Input: part model. Units: mm. Frame: model coordinates. A direction names the side the tool comes from. Coordinates: 2 decimals unless noted, no trailing zeros. Order: outer loops, then holes, each group sorted by start corner. A loop starts at its lowest first (then second) coordinate and runs counter-clockwise, first axis right, second up. Notation, with made-up numbers: (26, 17.5) - (50, 17.5) arc R23 ccw to (50, 49.5) - close; hole circle Ø9 at (58, 78.5). An arc over 180 degrees is marked (long way). Answer as CSV lines item,"result". Start each with the question number.
Item 1: Section B-B (y = -34.8). Output: boundary loops of the cut face in (x, z), and give its area (3 significant figures).
Item 2: Section A-A (z = -27.5). Output: boundary loops of the cut face in (x, y), and give its area (3 significant figures).
Item 3: Access query for faces 5 (the cylindrical face through (-27.903, 27.841, -38.594)), 6 (the cylindrical face through (-27.841, -27.903, -38.594)), 7 (the flat face through (37, 26.7, -39)), 8 (the flat face through (37, -26.7, -39)). Directions: +Z, -Z, +X, -X, +Y, -Y. A direction counts if a zero-diameter tool reaches every point of the face in a straight line with its end or side. Return the directions, or none.
Item 4: Section D-D (y = 0). Output: boundary loops of the cut face in (x, z).
Item 5: Draft query along Y for faces 1 (the cylindrical face through (-41.697, 41.759, -4.93)), 2 (the cylindrical face through (-38.022, -34.377, -5.07)), 3 (the cylindrical face through (6.466, 2.681, 16.587)), 4 (the flat face through (-26.7, -37, -39)). Return one class per face: +Y half, -Y half, draft (parallel to the pull), parting line (faces both ways), or undercut.
Item 6: First-contact query: pin 1 (5 mm diameter, centred on x = -35.5, y = -36.5, fed in from -Z); pin 2 (6 mm diameter, centred on x = -34.8, y = 34.8, fed in from +Z); pin 3 (2 mm diameter, centred on x = 4.5, y = 13.5, fed in from +Z); pin 4 (6 mm diameter, centred on y = 37, z = -31.5, fed in from +X). Flat tips, straight axial feed; report the tip coordinate or a pass-through.
Item 7: Material intervals for line 1 along Y through (x, z) = (34.8, -2.5); line 2 along X through (y, z) = (34, -2), sorted ascending.
Autodesk Inventor part; units mm, degrees
ref_plane "YZ Plane" through (0, 0, 0) normal (1, 0, 0) x (0, 1, 0)
ref_plane "XZ Plane" through (0, 0, 0) normal (0, 1, 0) x (-1, 0, 0)
ref_plane "XY Plane" through (0, 0, 0) normal (0, 0, 1) x (1, 0, 0)
sketch "Skizze1" plane through (0, 0, 0) normal (0, 0, 1) x (1, 0, 0)
  line L0 (-38.9, -42.9) -> (38.9, -42.9)
  line L1 (42.9, -38.9) -> (42.9, 38.9)
  line L2 (38.9, 42.9) -> (-38.9, 42.9)
  line L3 (-42.9, 38.9) -> (-42.9, -38.9)
  line L4 (-42.9, -42.9) -> (42.9, 42.9) construction
  line L5 (42.9, -42.9) -> (-42.9, 42.9) construction
  arc A0 (42.9, 38.9) -> (38.9, 42.9) centre (38.9, 38.9) ccw
  arc A1 (38.9, -42.9) -> (42.9, -38.9) centre (38.9, -38.9) ccw
  arc A2 (-42.9, -38.9) -> (-38.9, -42.9) centre (-38.9, -38.9) ccw
  arc A3 (-38.9, 42.9) -> (-42.9, 38.9) centre (-38.9, 38.9) ccw
  point P0 (0, 0)
  dimension "d0" = 4
  dimension "d1" = 85.8
extrude "Extrusion1" add sketch "Skizze1" against normal blind 10
sketch "Skizze2" plane through (0, 0, 0) normal (0, 0, 1) x (1, 0, 0)
  circle A0 centre (0, 0) radius 36.5
  dimension "d4" = 73
extrude "Extrusion2" add sketch "Skizze2" along normal blind 1.6
sketch "Skizze3" plane through (0, 0, -10) normal (0, 0, -1) x (-1, 0, 0)
  line L0 (-42.9, 38.9) -> (-42.9, -38.9)
  arc A0 (-42.9, -38.9) -> (-38.9, -42.9) centre (-38.9, -38.9) ccw
  line L1 (-38.9, -42.9) -> (38.9, -42.9)
  arc A1 (38.9, -42.9) -> (42.9, -38.9) centre (38.9, -38.9) ccw
  line L2 (42.9, -38.9) -> (42.9, 38.9)
  arc A2 (42.9, 38.9) -> (38.9, 42.9) centre (38.9, 38.9) ccw
  line L3 (38.9, 42.9) -> (-38.9, 42.9)
  arc A3 (-38.9, 42.9) -> (-42.9, 38.9) centre (-38.9, 38.9) ccw
  line L4 (42.9, -26.7) -> (30.7, -26.7)
  line L5 (26.7, -30.7) -> (26.7, -42.9)
  arc A4 (30.7, -26.7) -> (26.7, -30.7) centre (30.7, -30.7) ccw
  line L6 (38.9, -38.9) -> (-38.9, 38.9) construction
  circle A5 centre (34.8, -34.8) radius 8.1 construction
  line L7 (38.9, 38.9) -> (-38.9, -38.9) construction
  line L8 (34.8, -34.8) -> (-34.8, -34.8) construction
  line L9 (42.9, -38.9) -> (42.9, 38.9)
  line L10 (42.9, -26.7) -> (42.9, -38.9)
  line L11 (-38.9, -42.9) -> (38.9, -42.9)
  line L12 (26.7, -42.9) -> (38.9, -42.9)
  arc A6 (38.9, -42.9) -> (42.9, -38.9) centre (38.9, -38.9) ccw
  arc A7 (42.9, 38.9) -> (38.9, 42.9) centre (38.9, 38.9) ccw
  line L13 (42.9, 26.7) -> (42.9, 38.9)
  line L14 (30.7, 26.7) -> (42.9, 26.7)
  arc A8 (26.7, 30.7) -> (30.7, 26.7) centre (30.7, 30.7) ccw
  line L15 (26.7, 42.9) -> (26.7, 30.7)
  line L16 (26.7, 42.9) -> (38.9, 42.9)
  arc A9 (-38.9, 42.9) -> (-42.9, 38.9) centre (-38.9, 38.9) ccw
  line L17 (-26.7, 42.9) -> (-38.9, 42.9)
  line L18 (-26.7, 30.7) -> (-26.7, 42.9)
  arc A10 (-30.7, 26.7) -> (-26.7, 30.7) centre (-30.7, 30.7) ccw
  line L19 (-42.9, 26.7) -> (-30.7, 26.7)
  line L20 (-42.9, 26.7) -> (-42.9, 38.9)
  arc A11 (-42.9, -38.9) -> (-38.9, -42.9) centre (-38.9, -38.9) ccw
  line L21 (-42.9, -26.7) -> (-42.9, -38.9)
  line L22 (-30.7, -26.7) -> (-42.9, -26.7)
  arc A12 (-26.7, -30.7) -> (-30.7, -26.7) centre (-30.7, -30.7) ccw
  line L23 (-26.7, -42.9) -> (-26.7, -30.7)
  line L24 (-26.7, -42.9) -> (-38.9, -42.9)
  point P0 (0, 0)
  dimension "d7" = 4
  dimension "d8" = 69.6
  dimension "d11" = 360
extrude "Extrusion3" add sketch "Skizze3" along normal blind 58 contours L19 A10 L18 L3 L15 A8 L14 L2 L4 A4 L5 L1 L23 A12 L22 L0
sketch "Skizze4" plane through (0, 0, 0) normal (0, 0, 1) x (1, 0, 0)
  circle A0 centre (0, 0) radius 36.5
  line L0 (42.9, 38.9) -> (42.9, -38.9)
  arc A1 (42.9, 38.9) -> (38.9, 42.9) centre (38.9, 38.9) ccw
  line L1 (-38.9, 42.9) -> (38.9, 42.9)
  arc A2 (-38.9, 42.9) -> (-42.9, 38.9) centre (-38.9, 38.9) ccw
  line L2 (-42.9, -38.9) -> (-42.9, 38.9)
  arc A3 (-42.9, -38.9) -> (-38.9, -42.9) centre (-38.9, -38.9) ccw
  line L3 (38.9, -42.9) -> (-38.9, -42.9)
  arc A4 (38.9, -42.9) -> (42.9, -38.9) centre (38.9, -38.9) ccw
  line L4 (38.9, -38.9) -> (-38.9, 38.9) construction
  line L5 (-34.8, 34.8) -> (34.8, 34.8) construction
  line L6 (34.8, 34.8) -> (34.8, -34.8) construction
  line L7 (34.8, -34.8) -> (-34.8, -34.8) construction
  line L8 (-34.8, -34.8) -> (-34.8, 34.8) construction
  line L9 (-34.8, 34.8) -> (34.8, -34.8) construction
  line L10 (34.8, 34.8) -> (-34.8, -34.8) construction
  dimension "d15" = 69.6
hole "Bohrung1" at (34.8, 34.8, 0) at (-34.8, 34.8, 0) at (-34.8, -34.8, 0) at (34.8, -34.8, 0) direction (0, 0, -1) diameter 6.5 end through all
sketch "Skizze5" plane through (0, 0, 1.6) normal (0, 0, 1) x (1, 0, 0)
  circle A0 centre (0, 0) radius 7
  dimension "d23" = 14
extrude "Extrusion4" add sketch "Skizze5" along normal blind 30.4
properties part number "Nema34"
Determined:
1,outline,"(-42.9, -10) - (-38.05, -10) - (-38.05, 0) - (-42.9, 0) - close; (-31.55, -10) - (-26.7, -10) - (-26.7, -68) - (26.7, -68) - (26.7, -10) - (31.55, -10) - (31.55, 0) - (11.01, 0) - (11.01, 1.6) - (-11.01, 1.6) - (-11.01, 0) - (-31.55, 0) - close; (38.05, -10) - (42.9, -10) - (42.9, 0) - (38.05, 0) - close"
1,area,"3,860 mm^2"
2,outline,"(-42.9, -26.7) - (-30.7, -26.7) arc R4 cw to (-26.7, -30.7) - (-26.7, -42.9) - (26.7, -42.9) - (26.7, -30.7) arc R4 cw to (30.7, -26.7) - (42.9, -26.7) - (42.9, 26.7) - (30.7, 26.7) arc R4 cw to (26.7, 30.7) - (26.7, 42.9) - (-26.7, 42.9) - (-26.7, 30.7) arc R4 cw to (-30.7, 26.7) - (-42.9, 26.7) - close"
2,area,"6,330 mm^2"
3,face 5,"-Z, -X, +Y"
3,face 6,"-Z, -X, -Y"
3,face 7,"-Z, +X, +Y"
3,face 8,"-Z, +X, -Y"
4,outline,"(-42.9, -68) - (42.9, -68) - (42.9, 0) - (36.5, 0) - (36.5, 1.6) - (7, 1.6) - (7, 32) - (-7, 32) - (-7, 1.6) - (-36.5, 1.6) - (-36.5, 0) - (-42.9, 0) - close"
5,face 1,"+Y half"
5,face 2,"undercut"
5,face 3,"parting line"
5,face 4,"draft"
6,pin 1,"stops at z = -10"
6,pin 2,"passes through"
6,pin 3,"stops at z = 1.6"
6,pin 4,"stops at x = 26.7"
7,line 1,"y = -42.9 to -38.05, -31.55 to 31.55, 38.05 to 42.9"
7,line 2,"x = -42.9 to -37.95, -31.65 to 31.65, 37.95 to 42.9"
